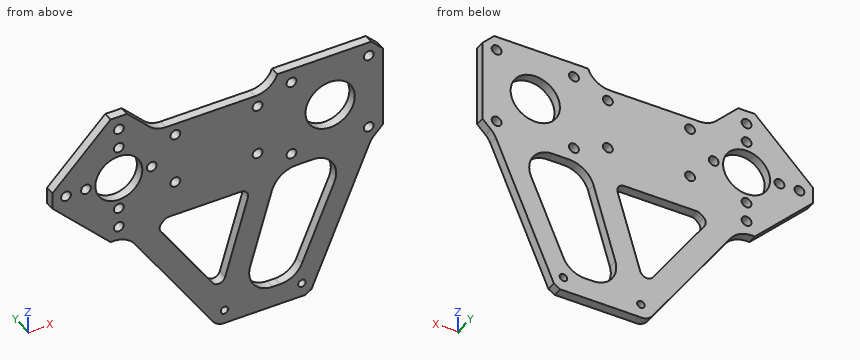
from build123d import *

# Parameters (mm, degrees)
SKETCH_1_R          = 2.1
SKETCH_1_R_2        = 10.5
SKETCH_1_R_3        = 10
EXTRUDE_1_DEPTH     = 4
CHAMFER_1_SIZE      = 5
FILLET_1_R          = 10
SKETCH_2_R          = 2.1
CUT_EXTRUDE_1_DEPTH = 10
EXTRUDE_START       = -4
SKETCH_3_R          = 1.6
EXTRUDE_2_DEPTH     = 4
FILLET_2_R          = 3
FILLET_3_R          = 11
SKETCH_4_R          = 1.6
EXTRUDE_3_DEPTH     = 4
FILLET_4_R          = 10
CHAMFER_2_SIZE      = 2
CHAMFER_2_SIZE2     = 1.851556395
FILLET_5_R          = 10


with BuildPart() as part:
    # 草图1 → 凸台-拉伸1 (new body)
    with BuildSketch(Plane(origin=(0, 0, 0), x_dir=(1, 0, 0), z_dir=(0, 1, 0))):
        Polygon((0, 31.819805153), (-31.819805153, 0), (0, -31.819805153), (15.909902577, -15.909902577), (67.5, -15.909902577), (67.5, -22.5), (112.5, -22.5), (112.5, 22.5), (67.5, 22.5), (67.5, 15.909902577), (15.909902577, 15.909902577), align=None)
        with Locations(Location((0, 14, 0), (0, 0, 270))):
            Circle(SKETCH_1_R, mode=Mode.SUBTRACT)
        with Locations(Location((14, 0, 0), (0, 0, 270))):
            Circle(SKETCH_1_R, mode=Mode.SUBTRACT)
        with Locations(Location((0, -14, 0), (0, 0, 270))):
            Circle(SKETCH_1_R, mode=Mode.SUBTRACT)
        with Locations(Location((-14, 0, 0), (0, 0, 270))):
            Circle(SKETCH_1_R, mode=Mode.SUBTRACT)
        with Locations(Location((90, 0, 0), (0, 0, 270))):
            Circle(SKETCH_1_R_2, mode=Mode.SUBTRACT)
        with Locations(Location((0, 22.5, 0), (0, 0, 270))):
            Circle(SKETCH_1_R, mode=Mode.SUBTRACT)
        with Locations(Location((0, -22.5, 0), (0, 0, 270))):
            Circle(SKETCH_1_R, mode=Mode.SUBTRACT)
        with Locations(Location((0, 0, 0), (0, 0, 270))):
            Circle(SKETCH_1_R_3, mode=Mode.SUBTRACT)
        with Locations(Location((-22.5, 0, 0), (0, 0, 270))):
            Circle(SKETCH_1_R, mode=Mode.SUBTRACT)
    extrude(amount=EXTRUDE_1_DEPTH)

    # 倒角1
    chamfer_1_edges = [part.edges().sort_by_distance(p)[0] for p in [
        (112.5, 2, -22.5),
        (112.5, 2, 22.5),
        (0, 2, 31.819805153),
        (-31.819805153, 2, 0),
        (0, 2, -31.819805153),
    ]]
    chamfer(chamfer_1_edges, length=CHAMFER_1_SIZE)

    # 圆角1
    # the kernel refuses this fillet: 10 mm, written as the material it adds along each edge
    with BuildSketch(Plane(origin=(15.909902577, 0, -15.909902577), x_dir=(-0.707106781186552, 0, -0.707106781186543), z_dir=(0, 1, 0))) as fillet_1_piece_1:
        with BuildLine():
            CenterArc((FILLET_1_R * 0.414213562373, -FILLET_1_R), FILLET_1_R, 90, 45)
            Line((-FILLET_1_R * 0.292893218813, -FILLET_1_R * 0.292893218813), (-FILLET_1_R * 0.307035354437, -FILLET_1_R * 0.27875108319))
            Line((-FILLET_1_R * 0.307035354437, -FILLET_1_R * 0.27875108319), (-FILLET_1_R * 0.00828427124746, FILLET_1_R * 0.02))
            Line((-FILLET_1_R * 0.00828427124746, FILLET_1_R * 0.02), (FILLET_1_R * 0.414213562373, FILLET_1_R * 0.02))
            Line((FILLET_1_R * 0.414213562373, FILLET_1_R * 0.02), (FILLET_1_R * 0.414213562373, 0))
        make_face()
    extrude(amount=4)
    with BuildSketch(Plane(origin=(15.909902577, 0, 15.909902577), x_dir=(-0.7071067811865422, 0, 0.707106781186553), z_dir=(0, 1, 0))) as fillet_1_piece_2:
        with BuildLine():
            CenterArc((FILLET_1_R * 0.414213562373, FILLET_1_R), FILLET_1_R, 225, 45)
            Line((-FILLET_1_R * 0.292893218813, FILLET_1_R * 0.292893218813), (-FILLET_1_R * 0.307035354437, FILLET_1_R * 0.27875108319))
            Line((-FILLET_1_R * 0.307035354437, FILLET_1_R * 0.27875108319), (-FILLET_1_R * 0.00828427124746, -FILLET_1_R * 0.02))
            Line((-FILLET_1_R * 0.00828427124746, -FILLET_1_R * 0.02), (FILLET_1_R * 0.414213562373, -FILLET_1_R * 0.02))
            Line((FILLET_1_R * 0.414213562373, -FILLET_1_R * 0.02), (FILLET_1_R * 0.414213562373, 0))
        make_face()
    extrude(amount=4)
    with BuildSketch(Plane(origin=(67.5, 0, 15.909902577), x_dir=(-1, 0, 0), z_dir=(0, 1, 0))) as fillet_1_piece_3:
        with BuildLine():
            CenterArc((9.400668296, 10), FILLET_1_R, 199.937217397, 70.062782603)
            Line((0, 6.590097423), (-0.188013366, 6.521899372))
            ThreePointArc((-0.188013366, 6.521899372), (-0.2, 3.295048712), (-0.2, 0))
            Line((-0.2, 0), (0, -0.2))
            Line((0, -0.2), (9.400668296, -0.2))
            Line((9.400668296, -0.2), (9.400668296, 0))
        make_face()
    extrude(amount=4)
    with BuildSketch(Plane(origin=(67.5, 0, -15.909902577), x_dir=(-1, 0, 0), z_dir=(0, 1, 0))) as fillet_1_piece_4:
        with BuildLine():
            CenterArc((9.400668296, -10), FILLET_1_R, 90, 70.062782603)
            Line((0, -6.590097423), (-0.188013366, -6.521899372))
            ThreePointArc((-0.188013366, -6.521899372), (-0.2, -3.295048712), (-0.2, 0))
            Line((-0.2, 0), (0, 0.2))
            Line((0, 0.2), (9.400668296, 0.2))
            Line((9.400668296, 0.2), (9.400668296, 0))
        make_face()
    extrude(amount=4)

    # 草图2 → 切除-拉伸1 (cut)
    with BuildSketch(Plane.XZ):
        with Locations(Location((106.464466094, 16.464466094, 0), (0, 0, 270))):
            Circle(SKETCH_2_R)
        with Locations(Location((106.464466094, -16.464466094, 0), (0, 0, 270))):
            Circle(SKETCH_2_R)
        with Locations(Location((73.535533906, -16.464466094, 0), (0, 0, 90))):
            Circle(SKETCH_2_R)
        with Locations(Location((73.535533906, 16.464466094, 0), (0, 0, 90))):
            Circle(SKETCH_2_R)
        with Locations(Location((24.075684952, 10.909902577, 0), (0, 0, 270))):
            Circle(SKETCH_2_R)
        with Locations(Location((59.075684952, 10.909902577, 0), (0, 0, 270))):
            Circle(SKETCH_2_R)
        with Locations(Location((59.075684952, -10.909902577, 0), (0, 0, 90))):
            Circle(SKETCH_2_R)
        with Locations(Location((24.075684952, -10.909902577, 0), (0, 0, 90))):
            Circle(SKETCH_2_R)
    extrude(amount=-CUT_EXTRUDE_1_DEPTH, mode=Mode.SUBTRACT)

    # 草图3 → 凸台-拉伸2 (add)
    with BuildSketch(Plane(origin=(0, 4, 0), x_dir=(1, 0, 0), z_dir=(0, 1, 0)).offset(EXTRUDE_START)):
        with BuildLine():
            Line((3.535533906, 28.284271247), (40.057636417, 81.344203773))
            ThreePointArc((40.057636417, 81.344203773), (45.94930127, 83.86671265), (50.75784592, 79.629654221))
            Line((50.75784592, 79.629654221), (67.5, 22.5))
            ThreePointArc((67.5, 22.5), (63.839583189, 17.721525883), (58.099331704, 15.909902577))
            Line((58.099331704, 15.909902577), (20.0520382, 15.909902577))
            ThreePointArc((20.0520382, 15.909902577), (16.225203877, 16.671107252), (12.980970389, 18.838834765))
            Line((12.980970389, 18.838834765), (3.535533906, 28.284271247))
        make_face()
        with Locations(Location((45, 77.942286341, 0), (0, 0, 270))):
            Circle(SKETCH_3_R, mode=Mode.SUBTRACT)
        Polygon((16.491758356, 29.470182421), (43.526560522, 68.746803428), (56.080145943, 25.909902577), (20.0520382, 25.909902577), align=None, mode=Mode.SUBTRACT)
    extrude(amount=EXTRUDE_2_DEPTH)

    # 圆角2
    fillet_2_edges = [part.edges().sort_by_distance(p)[0] for p in [
        (16.491758356, 2, -29.470182421),
        (43.526560522, 2, -68.746803428),
        (56.080145943, 2, -25.909902577),
        (20.0520382, 2, -25.909902577),
    ]]
    fillet(fillet_2_edges, radius=FILLET_2_R)

    # 圆角3
    fillet_3_edges = [part.edges().sort_by_distance(p)[0] for p in [
        (67.5, 2, -22.5),
        (3.535533906, 2, -28.284271247),
    ]]
    fillet(fillet_3_edges, radius=FILLET_3_R)

    # 草图4 → 凸台-拉伸3 (add)
    with BuildSketch(Plane(origin=(0, 4, 0), x_dir=(1, 0, 0), z_dir=(0, 1, 0)).offset(EXTRUDE_START)):
        with BuildLine():
            Line((45.94930127, 83.86671265), (81.347717681, 83.86671265))
            Line((81.347717681, 83.86671265), (107.5, 22.5))
            Line((107.5, 22.5), (97.716806526, 22.5))
            Line((97.716806526, 22.5), (75.4, 74.86671265))
            Line((75.4, 74.86671265), (52.153651701, 74.86671265))
            Line((52.153651701, 74.86671265), (50.75784592, 79.629654221))
            ThreePointArc((50.75784592, 79.629654221), (48.966689034, 82.443994695), (45.94930127, 83.86671265))
        make_face()
        with Locations(Location((78, 77.942286341, 0), (0, 0, 270))):
            Circle(SKETCH_4_R, mode=Mode.SUBTRACT)
    extrude(amount=EXTRUDE_3_DEPTH)

    # 圆角4
    fillet_4_edges = [part.edges().sort_by_distance(p)[0] for p in [
        (97.716806526, 2, -22.5),
        (75.4, 2, -74.86671265),
        (52.153651701, 2, -74.86671265),
    ]]
    fillet(fillet_4_edges, radius=FILLET_4_R)

    # 倒角2
    chamfer_2_edges = [part.edges().sort_by_distance(p)[0] for p in [
        (81.347717681, 2, -83.86671265),
    ]]
    chamfer_2_side = [part.faces().sort_by_distance(p)[0] for p in [
        (63.648509476, 2, -83.86671265),
    ]]
    chamfer(chamfer_2_edges, length=CHAMFER_2_SIZE, length2=CHAMFER_2_SIZE2, reference=chamfer_2_side[0])

    # 圆角5
    fillet_5_edges = [part.edges().sort_by_distance(p)[0] for p in [
        (107.5, 2, -22.5),
    ]]
    fillet(fillet_5_edges, radius=FILLET_5_R)


solid = part.part
Geometry check sheet. Reference: the model listing, model coordinates, mm. Coordinates: 2 decimals unless noted, no trailing zeros. Order: outer loops, then holes, each group sorted by start corner. A loop starts at its lowest first (then second) coordinate and runs counter-clockwise, first axis right, second up. Notation, with made-up numbers: (8, 3.5) - (25, 3.5) arc R22 ccw to (25, 34.5) - close; hole circle Ø2 at (71.25, -27). An arc over 180 degrees is marked (long way). One line per item, written item: value.
(1) Thickness scan on probe 1 along X at (y, z) = (1.4, 0); probe 2 along Z at (x, y) = (78, 2.1); probe 3 along Z at (x, y) = (-1.5, 3.8). Record the ranges inside material, lowest first. Write a range as from..to.
Data:
probe 1: x = -28.28..-24.6, -20.4..-16.1, -11.9..-10, 10..11.9, 16.1..79.5, 100.5..112.5
probe 2: z = -83.87..-79.54, -76.34..-68.77, -22.5..22.5
probe 3: z = -28.31..-23.97, -21.03..-15.47, -12.53..-9.89, 9.89..12.53, 15.47..21.03, 23.97..28.28
(2) Sectioned sample at A-A (z = 0). Enter the section's corners in (x, y).
Data:
outline: (-28.28, 0) - (-24.6, 0) - (-24.6, 4) - (-28.28, 4) - close; (-20.4, 0) - (-16.1, 0) - (-16.1, 4) - (-20.4, 4) - close; (-11.9, 0) - (-10, 0) - (-10, 4) - (-11.9, 4) - close; (10, 0) - (11.9, 0) - (11.9, 4) - (10, 4) - close; (16.1, 0) - (79.5, 0) - (79.5, 4) - (16.1, 4) - close; (100.5, 0) - (112.5, 0) - (112.5, 4) - (100.5, 4) - close
(3) Sectioned sample at C-C (x = -14). Enter the section's corners in (y, z), and give its area (3 significant figures).
Data:
outline: (0, -17.82) - (4, -17.82) - (4, -2.1) - (0, -2.1) - close; (0, 2.1) - (4, 2.1) - (4, 17.82) - (0, 17.82) - close
area: 126 mm^2
(4) Sectioned sample at B-B (z = -47). Enter the section's corners in (x, y), and give its area (3 significant figures).
Data:
outline: (16.42, 0) - (28.56, 0) - (28.56, 4) - (16.42, 4) - close; (49.9, 0) - (60.32, 0) - (60.32, 4) - (49.9, 4) - close; (87.28, 0) - (97.06, 0) - (97.06, 4) - (87.28, 4) - close
area: 129 mm^2
(5) Depth check by flat-ended pin: pin 1 Ø12 at (x, z) = (50.5, -41) entering from -Y; pin 2 Ø1.5 at (y, z) = (3.5, -15) entering from -X. Enter the tip coordinate at first touch or a pass-through.
Data:
pin 1: stops at y = 0
pin 2: stops at x = -17.57
(6) Sectioned sample at D-D (y = 2.4). Count the separate pieces of the cut face and the enclosed holes in it, and give its area (3 significant figures).
Data:
separate pieces: 1
enclosed holes: 21
area: 7,210 mm^2
